from build123d import *

# Parameters (mm, degrees)
IZIM2_W                      = 87
IZIM2_H                      = 110
Y_KSEKLIK_EKSTR_ZYON1_DEPTH  = 28
BO_ALTMA1_T                  = -2
IZIM3_W                      = 66
IZIM3_H                      = 10
KES_EKSTR_ZYON1_DEPTH        = 2
IZIM4_W                      = 14
IZIM4_H                      = 14
KES_EKSTR_ZYON3_DEPTH        = 110
IZIM5_W                      = 16
IZIM5_H                      = 110
Y_KSEKLIK_EKSTR_ZYON2_DEPTH  = 2
IZIM7_W                      = 10
IZIM7_H                      = 34
KES_EKSTR_ZYON4_DEPTH        = 1
IZIM8_W                      = 10
IZIM8_H                      = 4
IZIM8_W_2                    = 20
KES_EKSTR_ZYON5_DEPTH        = 2
IZIM9_W                      = 54
IZIM9_H                      = 10
KES_EKSTR_ZYON6_DEPTH        = 2
IZIM10_W                     = 87
IZIM10_H                     = 110
Y_KSEKLIK_EKSTR_ZYON4_DEPTH  = 2
IZIM11_W                     = 12
IZIM11_H                     = 10
KES_EKSTR_ZYON7_DEPTH        = 2
IZIM12_W                     = 2
IZIM12_H                     = 2
KES_EKSTR_ZYON8_DEPTH        = 2
IZIM14_W                     = 10
IZIM14_H                     = 34
KES_EKSTR_ZYON9_DEPTH        = 2
IZIM15_W                     = 106
IZIM15_H                     = 12
Y_KSEKLIK_EKSTR_ZYON15_DEPTH = 2


with BuildPart() as part:
    # Çizim2 → Yükseklik-Ekstrüzyon1 (new body)
    with BuildSketch(Plane(origin=(0, 0, 0), x_dir=(1, 0, 0), z_dir=(0, 1, 0))):
        with Locations((43.5, 55)):
            Rectangle(IZIM2_W, IZIM2_H)
    extrude(amount=Y_KSEKLIK_EKSTR_ZYON1_DEPTH)

    # İç Boşaltma1
    bo_altma1_openings = [part.faces().sort_by_distance(p)[0] for p in [
        (43.5, 28, -55),
        (43.5, 0, -55),
    ]]
    offset(amount=BO_ALTMA1_T, openings=bo_altma1_openings, kind=Kind.INTERSECTION)

    # Çizim3 → Kes-Ekstrüzyon1 (cut)
    with BuildSketch(Plane.ZY):
        with Locations((-73, 8.5)):
            Rectangle(IZIM3_W, IZIM3_H)
    extrude(amount=-KES_EKSTR_ZYON1_DEPTH, mode=Mode.SUBTRACT)

    # Çizim4 → Kes-Ekstrüzyon3 (cut)
    with BuildSketch(Plane(origin=(0, 0, -110), x_dir=(-1, 0, 0), z_dir=(0, 0, -1))):
        with Locations((-7, 21)):
            Rectangle(IZIM4_W, IZIM4_H)
    extrude(amount=-KES_EKSTR_ZYON3_DEPTH, mode=Mode.SUBTRACT)

    # Çizim5 → Yükseklik-Ekstrüzyon2 (add)
    with BuildSketch(Plane(origin=(0, 14, 0), x_dir=(1, 0, 0), z_dir=(0, 1, 0))):
        with Locations((8, 55)):
            Rectangle(IZIM5_W, IZIM5_H)
    extrude(amount=Y_KSEKLIK_EKSTR_ZYON2_DEPTH)

    # Çizim7 → Kes-Ekstrüzyon4 (cut)
    with BuildSketch(Plane(origin=(0, 16, 0), x_dir=(1, 0, 0), z_dir=(0, 1, 0))):
        with Locations((8, 20)):
            Rectangle(IZIM7_W, IZIM7_H)
    extrude(amount=-KES_EKSTR_ZYON4_DEPTH, mode=Mode.SUBTRACT)

    # Çizim8 → Kes-Ekstrüzyon5 (cut)
    with BuildSketch(Plane.XY):
        with Locations((25.500000105, 19)):
            Rectangle(IZIM8_W, IZIM8_H)
        with Locations((26, 15)):
            Rectangle(IZIM8_W_2, IZIM8_H)
    extrude(amount=-KES_EKSTR_ZYON5_DEPTH, mode=Mode.SUBTRACT)

    # Çizim9 → Kes-Ekstrüzyon6 (cut)
    with BuildSketch(Plane(origin=(87, 0, 0), x_dir=(0, 0, -1), z_dir=(1, 0, 0))):
        with Locations((30, 8.5)):
            Rectangle(IZIM9_W, IZIM9_H)
    extrude(amount=-KES_EKSTR_ZYON6_DEPTH, mode=Mode.SUBTRACT)

    # Çizim10 → Yükseklik-Ekstrüzyon4 (add)
    with BuildSketch(Plane.XZ):
        with Locations((43.5, -55)):
            Rectangle(IZIM10_W, IZIM10_H)
    extrude(amount=Y_KSEKLIK_EKSTR_ZYON4_DEPTH)

    # Çizim11 → Kes-Ekstrüzyon7 (cut)
    with BuildSketch(Plane(origin=(87, 0, 0), x_dir=(0, 0, -1), z_dir=(1, 0, 0))):
        with Locations((97, 8.5)):
            Rectangle(IZIM11_W, IZIM11_H)
    extrude(amount=-KES_EKSTR_ZYON7_DEPTH, mode=Mode.SUBTRACT)

    # Çizim12 → Kes-Ekstrüzyon8 (cut)
    with BuildSketch(Plane.XZ.offset(2)):
        with Locations((54, -6.5)):
            Rectangle(IZIM12_W, IZIM12_H)
        with Locations((54, -38.5)):
            Rectangle(IZIM12_W, IZIM12_H)
        with Locations((54, -22.5)):
            Rectangle(IZIM12_W, IZIM12_H)
        with Locations((54, -14.5)):
            Rectangle(IZIM12_W, IZIM12_H)
        with Locations((54, -30.5)):
            Rectangle(IZIM12_W, IZIM12_H)
    extrude(amount=-KES_EKSTR_ZYON8_DEPTH, mode=Mode.SUBTRACT)

    # Çizim14 → Kes-Ekstrüzyon9 (cut)
    with BuildSketch(Plane(origin=(0, 15, 0), x_dir=(1, 0, 0), z_dir=(0, 1, 0))):
        with Locations((8, 20)):
            Rectangle(IZIM14_W, IZIM14_H)
    extrude(amount=-KES_EKSTR_ZYON9_DEPTH, mode=Mode.SUBTRACT)

    # Çizim15 → Yükseklik-Ekstrüzyon15 (add)
    with BuildSketch(Plane.ZY.offset(-14)):
        with Locations((-55, 22)):
            Rectangle(IZIM15_W, IZIM15_H)
    extrude(amount=-Y_KSEKLIK_EKSTR_ZYON15_DEPTH)


solid = part.part
Geometry check sheet. Reference: the model listing, model coordinates, mm. A direction names the side the tool comes from. Round coordinates to 2 decimals unless told otherwise and drop trailing zeros. Loops run counter-clockwise (first coordinate to the right, second up) from the corner with the lowest first, then second, coordinate; pieces in that order, holes last. Notation, with made-up numbers: (10, 31) -> (22, 31) arc R24 cw to (22, 66) -> close; hole circle Ø8 at (31, 75.5). An arc over 180 degrees is marked (long way). Answer as a JSON object with one key per item and string values. Group by question number.
Item 1: Release check for a two-part mould opening along Z. For faces 1 (the face through (43, 13, -110)), 2 (the face through (43, 14, -108)), 3 (the face through (7, 16, -68)), 4 (the face through (9, 14, -68)) record: pulls with the +Z half, pulls with the -Z half, needs draft (parallel to the pull), parting line crosses it, or undercut.
Item 2: Cross-section at A-A, the plane z = -64. Record the cut outline in (x, y), plus the area to 3 significant figures.
Item 3: Set-up check for faces 5 (the face through (14, 22, -56)), 6 (the face through (43, 0, -54)), 7 (the face through (85.5, 28, -71.6)), 8 (the face through (53, 13, 0)), 9 (the face through (85, 17, -54)): record each of +Z, -Z, +X, -X, +Y, -Y from which the full face is reachable in a straight line by a thin tool's end or side.
Item 4: Thickness scan on line 1 along X through (y, z) = (15.5, -28); line 2 along Z through (x, y) = (30, 6.5); line 3 along X through (y, z) = (23.5, -42). Record the ranges inside material, lowest first.
Item 5: Cross-section at B-B, the plane y = 2.25. Record the cut outline in (x, z).
Item 6: Cross-section at D-D, the plane x = 9. Record the cut outline in (y, z), plus the area to 3 significant figures.
Item 7: Cross-section at C-C, the plane x = 33. Record the cut outline in (y, z).
Item 8: Depth check by flat-ended pin: pin 1 Ø1 at (x, z) = (48.5, -26.5) entering from +Y; pin 2 Ø0.6 at (x, z) = (1.5, -63.5) entering from +Y. Enter the tip coordinate at first touch or a pass-through.
Determined:
{
 "1": {"face 1": "pulls with the -Z half", "face 2": "undercut", "face 3": "needs draft", "face 4": "undercut"},
 "2": {"outline": "(0, -2) -> (87, -2) -> (87, 28) -> (85, 28) -> (85, 0) -> (2, 0) -> (2, 3.5) -> (0, 3.5) -> close; (0, 13.5) -> (2, 13.5) -> (2, 14) -> (16, 14) -> (16, 28) -> (14, 28) -> (14, 16) -> (0, 16) -> close", "area": "294 mm²"},
 "3": {"face 5": "+Z, -Z, -X, +Y", "face 6": "none", "face 7": "+Z, -Z, +X, -X, +Y", "face 8": "+Z, +X, -X, +Y, -Y", "face 9": "+Y"},
 "4": {"line 1": "x = 0 to 3, 13 to 16, 85 to 87", "line 2": "z = -110 to -108, -2 to 0", "line 3": "x = 14 to 16, 85 to 87"},
 "5": {"outline": "(0, -110) -> (87, -110) -> (87, 0) -> (0, 0) -> close; hole (2, -108) -> (85, -108) -> (85, -2) -> (2, -2) -> close"},
 "6": {"outline": "(-2, -110) -> (16, -110) -> (16, -37) -> (14, -37) -> (14, -108) -> (0, -108) -> (0, -2) -> (14, -2) -> (14, -3) -> (16, -3) -> (16, 0) -> (-2, 0) -> close", "area": "428 mm²"},
 "7": {"outline": "(-2, -110) -> (28, -110) -> (28, -108) -> (0, -108) -> (0, -2) -> (13, -2) -> (13, 0) -> (-2, 0) -> close; (17, -2) -> (28, -2) -> (28, 0) -> (17, 0) -> close"},
 "8": {"pin 1": "stops at y = 0", "pin 2": "stops at y = 16"}
}
